Source: three-view drawing plus pictorial views. Frame: mm from the lowest corner of the part. Round coordinates to 2 decimals unless told otherwise and drop trailing zeros. Order: outer loops, then holes, each group sorted by start corner. A loop starts at its lowest first (then second) coordinate and runs counter-clockwise, first axis right, second up. Notation, with made-up numbers: (32.5, 48) -> (68.5, 48) arc R37 cw to (68.5, 85) -> close; hole circle Ø1 at (65, 70.5). An arc over 180 degrees is marked (long way). Use a Markdown table: item, result.
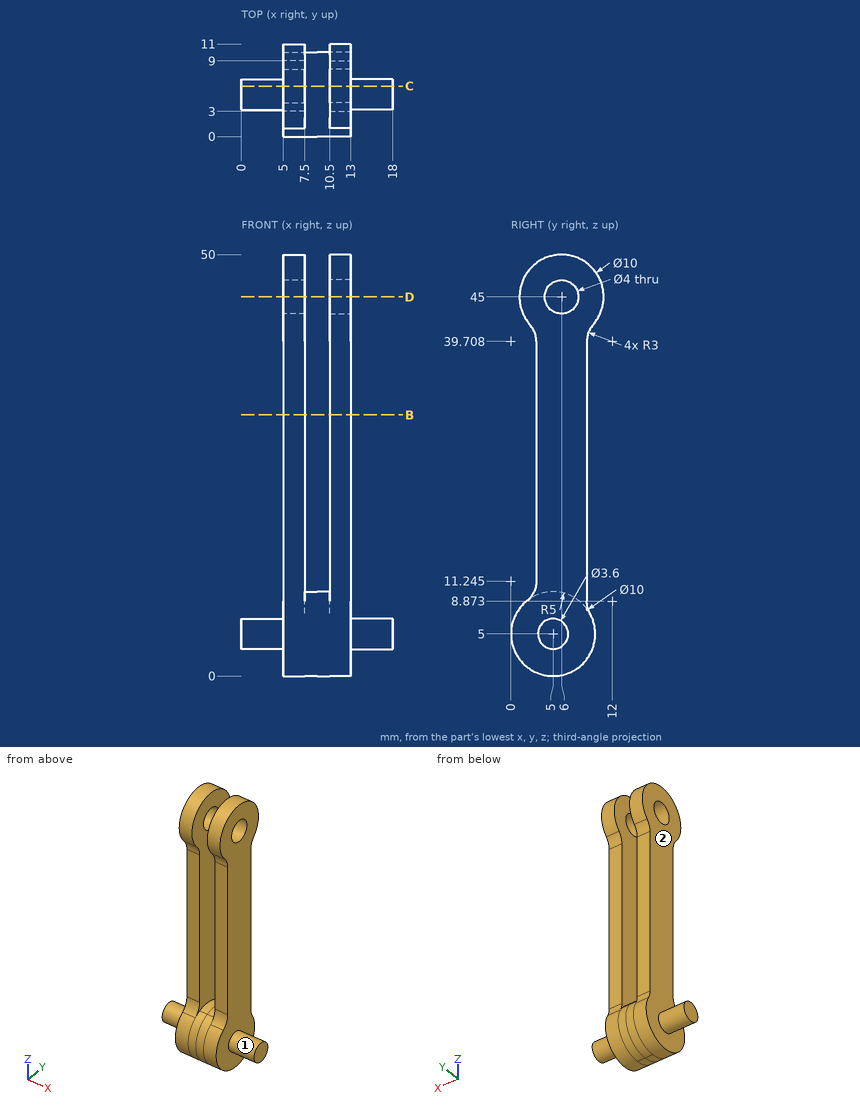
1) Cut plane C-C on y = 6. Return loops of the section in (x, z).
Results found:
| item | result |
|---|---|
| outline | (0, 3.5) -> (5, 3.5) -> (5, 0.1) -> (13, 0.1) -> (13, 3.5) -> (18, 3.5) -> (18, 6.5) -> (13, 6.5) -> (13, 43) -> (10.5, 43) -> (10.5, 9.9) -> (7.5, 9.9) -> (7.5, 43) -> (5, 43) -> (5, 6.5) -> (0, 6.5) -> close; (5, 47) -> (7.5, 47) -> (7.5, 50) -> (5, 50) -> close; (10.5, 47) -> (13, 47) -> (13, 50) -> (10.5, 50) -> close |
2) Line query: L1, parallel to Y at x = 11.4, z = 45; L2, parallel to X at y = 8.5, z = 40; L3, parallel to Y at x = 12.75, z = 31.5. Output: solid intervals per line, ascending. Write a range as [from, to].
Results found:
| item | result |
|---|---|
| L1 | y = [1, 4], [8, 11] |
| L2 | x = [5, 7.5], [10.5, 13] |
| L3 | y = [3, 9] |
3) Cut plane D-D on z = 45. Return loops of the section in (x, y).
Results found:
| item | result |
|---|---|
| outline | (5, 1) -> (7.5, 1) -> (7.5, 4) -> (5, 4) -> close; (5, 8) -> (7.5, 8) -> (7.5, 11) -> (5, 11) -> close; (10.5, 1) -> (13, 1) -> (13, 4) -> (10.5, 4) -> close; (10.5, 8) -> (13, 8) -> (13, 11) -> (10.5, 11) -> close |
4) Cut plane B-B on z = 31. Return loops of the section in (x, y), and give its area (3 significant figures).
Results found:
| item | result |
|---|---|
| outline | (5, 3) -> (7.5, 3) -> (7.5, 9) -> (5, 9) -> close; (10.5, 3) -> (13, 3) -> (13, 9) -> (10.5, 9) -> close |
| area | 30.0 mm² |
5) Pin query (flat end, axial travel): pin 1 Ø0.8 at (x, z) = (11, 21) entering from -Y; pin 2 Ø3.5 at (y, z) = (4.5, 33.5) entering from +X; pin 3 Ø1 at (y, z) = (5, 28) entering from -X; pin 4 Ø3 at (y, z) = (6, 45) entering from -X. Return the tip coordinate at first contact, or that it passes through.
Results found:
| item | result |
|---|---|
| pin 1 | stops at y = 3 |
| pin 2 | stops at x = 13 |
| pin 3 | stops at x = 5 |
| pin 4 | passes through |
6) Pull-direction query (Z, two-part tool) for the marked faces 1 and 2; classes: +Z half, -Z half, draft (parallel to the pull), parting line (faces both ways), or undercut.
Results found:
| item | result |
|---|---|
| face 1 | parting line |
| face 2 | draft |
